Input: part model. Units: mm. Frame: model coordinates. A direction names the side the tool comes from. Coordinates: 2 decimals unless noted, no trailing zeros. Write each loop counter-clockwise with the first axis right and the second up, starting at its lowest first coordinate (ties: lowest second). Pieces come first, ordered by that corner, then holes. Notation, with made-up numbers: (85.5, 24) - (111.5, 24) arc R30 cw to (111.5, 54) - close; hole circle Ø5 at (78, 69). An arc over 180 degrees is marked (long way). Put each result on its own line as item: value. Start each with the question number.
1. Access query for faces 1 (the flat face through (-1, -266, 16)), 2 (the flat face through (0, -266, 0)), 3 (the flat face through (1, -266, 16)). Directions: +Z, -Z, +X, -X, +Y, -Y. A direction counts if a zero-diameter tool reaches every point of the face in a straight line with its end or side. Return the directions, or none.
2. Cut plane A-A, the plane y = -459. Return loops of the section in (x, z).
3. Cut plane C-C, the plane z = 16. Return loops of the section in (x, y).
4. Pin query (flat end, axial travel): pin 1 (10 mm diameter, centred on x = 10.5, y = -488, fed in from +Z); pin 2 (1 mm diameter, centred on x = -0.5, z = 18, fed in from +Y); pin 3 (5 mm diameter, centred on y = -114, z = 7.5, fed in from -X). Return the tip coordinate at first contact, or that it passes through.
5. Cut plane B-B, the plane x = -8.75. Return loops of the section in (y, z), and give its area (3 significant figures).
6. Line query: line 1 (X direction, y = -460.5, z = 12); line 2 (Z direction, x = -6.5, y = -171.5); line 3 (Y direction, x = 0.5, z = 19.25). Output: solid intervals per line, ascending.
from build123d import *

# Parameters (mm, degrees)
F1_DEPTH = 540
F3_DEPTH = 20
F5_DEPTH = 20


with BuildPart() as f1:
    # F0 (on Front) → F1 (new body)
    with BuildSketch(Plane.XZ):
        Polygon((1, 30), (0, 30), (-1, 30), (-1, 2), (-15, 2), (-15, 0), (0, 0), (15, 0), (15, 2), (1, 2), align=None)
    extrude(amount=F1_DEPTH)

    # F2 (on face) → F3 (join)
    with BuildSketch(Plane(origin=(0, 0, 0), x_dir=(-1, 0, 0), z_dir=(0, 1, 0))):
        Polygon((-1, 2), (-15, 2), (-15, 0), (15, 0), (15, 2), (1, 2), align=None)
    extrude(amount=F3_DEPTH)

    # F4 (on face) → F5 (join)
    with BuildSketch(Plane.XZ.offset(540)):
        Polygon((-1, 2), (-15, 2), (-15, 0), (15, 0), (15, 2), (1, 2), align=None)
    extrude(amount=F5_DEPTH)


solid = f1.part
Report:
1. face 1: +Z, -X, +Y, -Y
1. face 2: -Z, +X, -X, +Y, -Y
1. face 3: +Z, +X, +Y, -Y
2. outline: (-15, 0) - (15, 0) - (15, 2) - (1, 2) - (1, 30) - (-1, 30) - (-1, 2) - (-15, 2) - close
3. outline: (-1, -540) - (1, -540) - (1, 0) - (-1, 0) - close
4. pin 1: stops at z = 2
4. pin 2: stops at y = 0
4. pin 3: stops at x = -1
5. outline: (-560, 0) - (20, 0) - (20, 2) - (-560, 2) - close
5. area: 1,160 mm^2
6. line 1: x = -1 to 1
6. line 2: z = 0 to 2
6. line 3: y = -540 to 0
